The listing builds one solid part. Answer for the finished solid, in the listing's coordinates (mm). Coordinates: 2 decimals unless noted, no trailing zeros. Order: outer loops, then holes, each group sorted by start corner. A loop starts at its lowest first (then second) coordinate and runs counter-clockwise, first axis right, second up. Notation, with made-up numbers: (43.5, 54) -> (60.5, 54) arc R16 cw to (60.5, 63) -> close; hole circle Ø3 at (-29, -9). An arc over 180 degrees is marked (long way). Return JSON: item names as keys, results as strings.
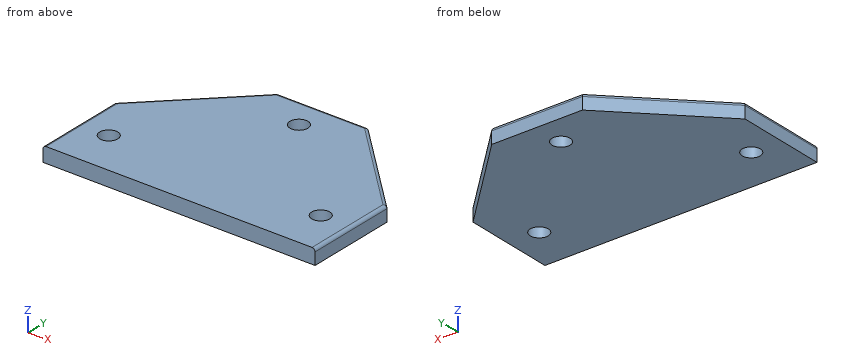
from build123d import *

# Parameters (mm, degrees)
BOSS_EXTRUDE1_DEPTH = 6.35
FILLET1_R           = 1.27
SKETCH3_R           = 3.81
CUT_EXTRUDE1_DEPTH  = 6.35


with BuildPart() as part:
    # Sketch1 → Boss-Extrude1 (new body)
    with BuildSketch(Plane.XY):
        Polygon((0, 38.1), (38.1, 76.2), (76.2, 76.2), (114.3, 38.1), (114.3, 0), (0, 0), align=None)
    extrude(amount=BOSS_EXTRUDE1_DEPTH)

    # Fillet1
    fillet1_edges = [part.edges().sort_by_distance(p)[0] for p in [
        (114.3, 19.05, 6.35),
        (95.25, 57.15, 6.35),
        (57.15, 76.2, 6.35),
        (19.05, 57.15, 6.35),
        (0, 19.05, 6.35),
    ]]
    fillet(fillet1_edges, radius=FILLET1_R)

    # Sketch3 → Cut-Extrude1 (cut)
    with BuildSketch(Plane.XY.offset(6.35)):
        with Locations((12.7, 18.813572483)):
            Circle(SKETCH3_R)
        with Locations((101.6, 19.02044656)):
            Circle(SKETCH3_R)
        with Locations((57.15, 63.5)):
            Circle(SKETCH3_R)
    extrude(amount=-CUT_EXTRUDE1_DEPTH, mode=Mode.SUBTRACT)


solid = part.part
1. Consider line 1 (Y direction, x = 57.15, z = 2); line 2 (X direction, y = 22, z = 1); line 3 (Y direction, x = 101.6, z = 2.25). Determine where each line is inside the solid, lowest interval first. Write a range as from..to.
Answer block:
{"line 1": "y = 0..59.69, 67.31..76.2", "line 2": "x = 0..10.61, 14.79..99.23, 103.97..114.3", "line 3": "y = 0..15.21, 22.83..50.8"}
2. Each of these flat-tipped pins is pushed along its axis until it touches: pin 1 Ø4 at (x, y) = (16.5, 59.5) entering from +Z (3 decimals); pin 2 Ø2 at (y, z) = (58.5, 4) entering from -X. Where does it stop, or does it pass through?
Answer block:
{"pin 1": "passes through", "pin 2": "stops at x = 19.4"}
3. The part is cut by section A-A on x = 57.15. Give the vertices of the cut face in (y, z).
Answer block:
{"outline": "(0, 0) -> (59.69, 0) -> (59.69, 6.35) -> (0, 6.35) -> close; (67.31, 0) -> (76.2, 0) -> (76.2, 5.08) arc R1.27 ccw to (74.93, 6.35) -> (67.31, 6.35) -> close"}
4. The part is cut by section B-B on z = 3.75. Give the vertices of the cut face in (x, y), and give its area (3 significant figures).
Answer block:
{"outline": "(0, 0) -> (114.3, 0) -> (114.3, 38.1) -> (76.2, 76.2) -> (38.1, 76.2) -> (0, 38.1) -> close; hole circle Ø7.62 at (12.7, 18.81); hole circle Ø7.62 at (57.15, 63.5); hole circle Ø7.62 at (101.6, 19.02)", "area": "7,120 mm2"}
